Geometry check sheet. Reference: the model listing, model coordinates, mm. Face numbers are marked on the shaded views. A direction names the side the tool comes from. Give positions to 0.01 mm unless a question says otherwise; leave off trailing zeros. Loops run counter-clockwise (first coordinate to the right, second up) from the corner with the lowest first, then second, coordinate; pieces in that order, holes last.
1. Cross-section at B-B, the plane x = -18. Record the cut outline in (y, z), plus the area to 3 significant figures.
2. Cross-section at A-A, the plane z = 0.45. State how many separate pieces and enclosed holes the cut face has, plus the area to 3 significant figures.
3. Cross-section at D-D, the plane x = 2. Record the cut outline in (y, z), plus the area to 3 significant figures.
4. Cross-section at C-C, the plane y = 1.75. Record the cut outline in (x, z).
5. Go/stop test with flat-tipped pins: pin 1 Ø1.5 at (x, y) = (4.5, 1.5) entering from +Z; pin 2 Ø3 at (x, y) = (17.5, 0) entering from -Z; pin 3 Ø2 at (y, z) = (-2, 1.5) entering from +X. Record where each tip stops, or that it passes through.
6. Release check for a two-part mould opening along Y. For the marked faces 3, 4 and 5 record: +Y half, -Y half, draft (parallel to the pull), parting line (faces both ways), or undercut.
7. Material ranges on L1, parallel to Y at x = 17.5, z = 2.7; L2, parallel to X at y = 0.5, z = 2.4; L3, parallel to Z at x = 9, y = -2.5, recorded low to high.
8. Tool access check on the marked faces 1 and 2. Record the directions out of +Z, -Z, +X, -X, +Y, -Y that give a thin tool (end or side, any length) a straight path to the whole face; none if there is none.
from build123d import *

# Parameters (mm, degrees)
SKETCH1_W               = 41
SKETCH1_H               = 6
SKETCH1_R               = 1.3
BOSS_EXTRUDE1_DEPTH     = 4
FILLET1_R               = 3
CUT_EXTRUDE1_DEPTH      = 22.731313812
CUT_EXTRUDE1_DEPTH_BACK = 22.731313812
FILLET2_R               = 3


with BuildPart() as part:
    # Sketch1 → Boss-Extrude1 (new body)
    with BuildSketch(Plane.XY):
        Rectangle(SKETCH1_W, SKETCH1_H)
        with Locations((17.5, 0)):
            Circle(SKETCH1_R, mode=Mode.SUBTRACT)
        with Locations((-17.5, 0)):
            Circle(SKETCH1_R, mode=Mode.SUBTRACT)
    extrude(amount=BOSS_EXTRUDE1_DEPTH)

    # Fillet1
    fillet1_edges = [part.edges().sort_by_distance(p)[0] for p in [
        (-20.5, -3, 2),
        (-20.5, 3, 2),
        (20.5, -3, 2),
        (20.5, 3, 2),
    ]]
    fillet(fillet1_edges, radius=FILLET1_R - 0.0001)  # a hair under: the kernel refuses the full size

    # Sketch2 → Cut-Extrude1 (cut, two sides: drawn at the far end of the back side and taken through both)
    with BuildSketch(Plane.XZ.offset(3).offset(-CUT_EXTRUDE1_DEPTH_BACK)):
        Polygon((-70.188274573, 60.188274573), (-14, 4), (-11, 1), (11, 1), (14, 4), (70.188274573, 60.188274573), (70.188274573, 219.112714467), (-70.188274573, 219.112714467), align=None)
    extrude(amount=CUT_EXTRUDE1_DEPTH + CUT_EXTRUDE1_DEPTH_BACK, mode=Mode.SUBTRACT)

    # Fillet2
    fillet2_edges = [part.edges().sort_by_distance(p)[0] for p in [
        (-11, 0, 1),
        (11, 0, 1),
        (14, 0, 4),
        (-14, 0, 4),
    ]]
    fillet(fillet2_edges, radius=FILLET2_R)


solid = part.part
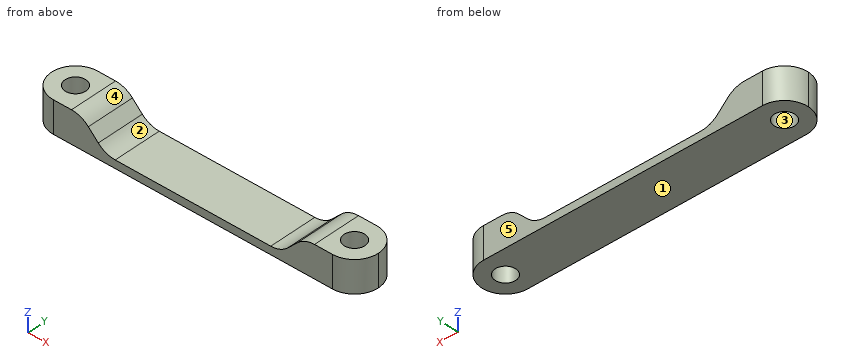
Result:
1. outline: (-2.96, 0) - (-1.2, 0) - (-1.2, 4) - (-2.96, 4) - close; (1.2, 0) - (2.96, 0) - (2.96, 4) - (1.2, 4) - close
1. area: 14.1 mm2
2. separate pieces: 1
2. enclosed holes: 2
2. area: 228 mm2
3. outline: (-3, 0) - (3, 0) - (3, 1) - (-3, 1) - close
3. area: 6.00 mm2
4. outline: (-19.94, 0) - (19.94, 0) - (19.94, 4) - (15.24, 4) arc R3 ccw to (13.12, 3.12) - (11.88, 1.88) arc R3 cw to (9.76, 1) - (-9.76, 1) arc R3 cw to (-11.88, 1.88) - (-13.12, 3.12) arc R3 ccw to (-15.24, 4) - (-19.94, 4) - close
5. pin 1: stops at z = 1
5. pin 2: stops at z = 0
5. pin 3: stops at x = 20.33
6. face 3: undercut
6. face 4: draft
6. face 5: +Y half
7. L1: y = -3 to -1.3, 1.3 to 3
7. L2: x = -20.46 to -18.7, -16.3 to -12.4, 12.4 to 16.3, 18.7 to 20.46
7. L3: z = 0 to 1
8. face 1: -Z, +X, -X, +Y, -Y
8. face 2: +Z, +Y, -Y
